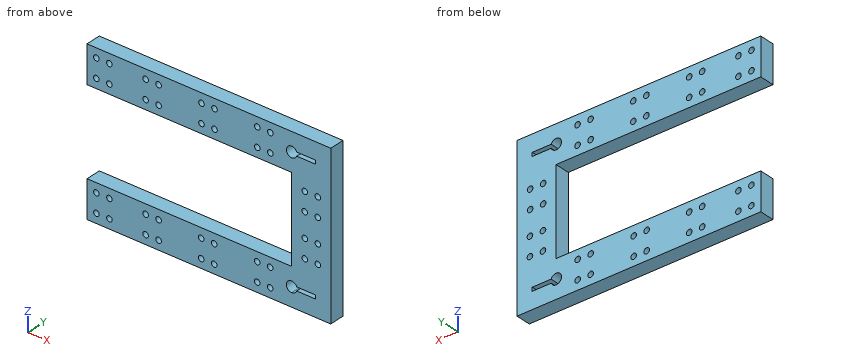
from build123d import *

# Parameters (mm, degrees)
SKETCH1_R           = 1.5
BOSS_EXTRUDE1_DEPTH = 8


with BuildPart() as part:
    # Sketch1 → Boss-Extrude1 (new body)
    with BuildSketch(Plane(origin=(0, 0, 0), x_dir=(1, 0, 0), z_dir=(0, 1, 0))):
        Polygon((21, 42.996794864), (21, 22.996794864), (130.982222222, 22.996794864), (130.982222222, -23.003205136), (20.982222222, -23.003205136), (20.982222222, -43.003205136), (151.982222222, -43.003205136), (151.982222222, 42.996794864), align=None)
        with BuildLine():
            ThreePointArc((133.652222222, -34), (128.132224278, -33.006627887), (133.649820291, -32))
            Line((133.649820291, -32), (143.832222222, -32))
            Line((143.832222222, -32), (143.832222222, -34))
            Line((143.832222222, -34), (133.652222222, -34))
        make_face(mode=Mode.SUBTRACT)
        with Locations((25.982222222, -38.003205136)):
            Circle(SKETCH1_R, mode=Mode.SUBTRACT)
        with Locations((32.982222222, -38.003205136)):
            Circle(SKETCH1_R, mode=Mode.SUBTRACT)
        with Locations((52.447128478, -37.978244052)):
            Circle(SKETCH1_R, mode=Mode.SUBTRACT)
        with Locations((59.447128478, -37.978244052)):
            Circle(SKETCH1_R, mode=Mode.SUBTRACT)
        with Locations((82.483268969, -37.971182344)):
            Circle(SKETCH1_R, mode=Mode.SUBTRACT)
        with Locations((89.483268969, -37.971182344)):
            Circle(SKETCH1_R, mode=Mode.SUBTRACT)
        with Locations((112.466817988, -38.005600575)):
            Circle(SKETCH1_R, mode=Mode.SUBTRACT)
        with Locations((119.466817988, -38.005600575)):
            Circle(SKETCH1_R, mode=Mode.SUBTRACT)
        with Locations((137.961991401, -16.468728947)):
            Circle(SKETCH1_R, mode=Mode.SUBTRACT)
        with Locations((144.961991401, -16.468728947)):
            Circle(SKETCH1_R, mode=Mode.SUBTRACT)
        with Locations((137.961991401, -6.468728947)):
            Circle(SKETCH1_R, mode=Mode.SUBTRACT)
        with Locations((144.961991401, -6.468728947)):
            Circle(SKETCH1_R, mode=Mode.SUBTRACT)
        with Locations((26, 27.996794864)):
            Circle(SKETCH1_R, mode=Mode.SUBTRACT)
        with Locations((33, 27.996794864)):
            Circle(SKETCH1_R, mode=Mode.SUBTRACT)
        with Locations((52.451959098, 28.108564772)):
            Circle(SKETCH1_R, mode=Mode.SUBTRACT)
        with Locations((26, 37.996794864)):
            Circle(SKETCH1_R, mode=Mode.SUBTRACT)
        with Locations((33, 37.996794864)):
            Circle(SKETCH1_R, mode=Mode.SUBTRACT)
        with Locations((52.451959098, 38.108564772)):
            Circle(SKETCH1_R, mode=Mode.SUBTRACT)
        with Locations((59.451959098, 28.108564772)):
            Circle(SKETCH1_R, mode=Mode.SUBTRACT)
        with Locations((82.310079685, 28.153226863)):
            Circle(SKETCH1_R, mode=Mode.SUBTRACT)
        with Locations((59.451959098, 38.108564772)):
            Circle(SKETCH1_R, mode=Mode.SUBTRACT)
        with Locations((82.310079685, 38.153226863)):
            Circle(SKETCH1_R, mode=Mode.SUBTRACT)
        with Locations((138.044723892, 6.53090338)):
            Circle(SKETCH1_R, mode=Mode.SUBTRACT)
        with Locations((145.044723892, 6.53090338)):
            Circle(SKETCH1_R, mode=Mode.SUBTRACT)
        with Locations((138.044723892, 16.53090338)):
            Circle(SKETCH1_R, mode=Mode.SUBTRACT)
        with Locations((145.044723892, 16.53090338)):
            Circle(SKETCH1_R, mode=Mode.SUBTRACT)
        with Locations((89.310079685, 28.153226863)):
            Circle(SKETCH1_R, mode=Mode.SUBTRACT)
        with Locations((112.409987019, 27.931087325)):
            Circle(SKETCH1_R, mode=Mode.SUBTRACT)
        with Locations((89.310079685, 38.153226863)):
            Circle(SKETCH1_R, mode=Mode.SUBTRACT)
        with Locations((112.409987019, 37.931087325)):
            Circle(SKETCH1_R, mode=Mode.SUBTRACT)
        with Locations((119.409987019, 27.931087325)):
            Circle(SKETCH1_R, mode=Mode.SUBTRACT)
        with Locations((119.409987019, 37.931087325)):
            Circle(SKETCH1_R, mode=Mode.SUBTRACT)
        with BuildLine():
            ThreePointArc((130.982222222, 35.864572641), (132.618738584, 35.351781823), (133.67, 33.996794864))
            Line((133.67, 33.996794864), (143.85, 33.996794864))
            Line((143.85, 33.996794864), (143.85, 31.996794864))
            Line((143.85, 31.996794864), (133.67, 31.996794864))
            ThreePointArc((133.67, 31.996794864), (128.627235263, 31.360278502), (130.982222222, 35.864572641))
        make_face(mode=Mode.SUBTRACT)
        with Locations((52.447128478, -27.978244052)):
            Circle(SKETCH1_R, mode=Mode.SUBTRACT)
        with Locations((59.447128478, -27.978244052)):
            Circle(SKETCH1_R, mode=Mode.SUBTRACT)
        with Locations((82.483268969, -27.971182344)):
            Circle(SKETCH1_R, mode=Mode.SUBTRACT)
        with Locations((89.483268969, -27.971182344)):
            Circle(SKETCH1_R, mode=Mode.SUBTRACT)
        with Locations((112.466817988, -28.005600575)):
            Circle(SKETCH1_R, mode=Mode.SUBTRACT)
        with Locations((119.466817988, -28.005600575)):
            Circle(SKETCH1_R, mode=Mode.SUBTRACT)
        with Locations((25.982222222, -28.003205136)):
            Circle(SKETCH1_R, mode=Mode.SUBTRACT)
        with Locations((32.982222222, -28.003205136)):
            Circle(SKETCH1_R, mode=Mode.SUBTRACT)
    extrude(amount=BOSS_EXTRUDE1_DEPTH)


solid = part.part
The listing builds one solid part. Answer for the finished solid, in the listing's coordinates (mm). Give positions to 0.01 mm unless a question says otherwise; leave off trailing zeros. Write each loop counter-clockwise with the first axis right and the second up, starting at its lowest first coordinate (ties: lowest second). Pieces come first, ordered by that corner, then holes.
Item 1: A flat-ended cylindrical pin translates along its axis: P1, Ø4, axis at y = 4, z = -34, coming from the -X side. Find the tip coordinate at first contact, or state that the pin passes through.
Item 2: Section C-C, the plane y = 5.5 is taken. Count the separate pieces of the cut face and the enclosed holes in it, plus the area to 3 significant figures.
Item 3: Find the intervals of material crossed by line 1 along Z through (x, y) = (143, 2.75); line 2 along Z through (x, y) = (121.5, 4); line 3 along X through (y, z) = (5.25, 16), in increasing order.
Item 4: Section B-B, the plane z = -19.5 is taken. Write down the section's boundary in (x, y), plus the area to 3 significant figures.
Item 5: Section A-A, the plane x = 33 is taken. Write down the section's boundary in (y, z), plus the area to 3 significant figures.
Completed:
1. P1: stops at x = 21
2. separate pieces: 1
2. enclosed holes: 42
2. area: 5,830 mm2
3. line 1: z = -43 to -34, -32 to 32, 34 to 43
3. line 2: z = -43 to -23, 23 to 43
3. line 3: x = 130.98 to 136.54, 139.39 to 143.54, 146.39 to 151.98
4. outline: (130.98, 0) - (151.98, 0) - (151.98, 8) - (130.98, 8) - close
4. area: 168 mm2
5. outline: (0, -43) - (8, -43) - (8, -39.5) - (0, -39.5) - close; (0, -36.5) - (8, -36.5) - (8, -29.5) - (0, -29.5) - close; (0, -26.5) - (8, -26.5) - (8, -23) - (0, -23) - close; (0, 23) - (8, 23) - (8, 26.5) - (0, 26.5) - close; (0, 29.5) - (8, 29.5) - (8, 36.5) - (0, 36.5) - close; (0, 39.5) - (8, 39.5) - (8, 43) - (0, 43) - close
5. area: 224 mm2
